Design review of the part built by this model. Coordinates are the model's own, in mm. A direction names the side the tool comes from. Give positions to 0.01 mm unless a question says otherwise; leave off trailing zeros. Loops run counter-clockwise (first coordinate to the right, second up) from the corner with the lowest first, then second, coordinate; pieces in that order, holes last. Notation, with made-up numbers: M 23,36 L 35,36 A22 ccw 35,73 Z; hole C 32.25,-31.75 d7. An arc over 180 degrees is marked long. Answer as CSV lines item,"result".
```python
from build123d import *

# Parameters (mm, degrees)
SKETCH1_R           = 45.25
SKETCH1_R_2         = 38.25
BOSS_EXTRUDE1_DEPTH = 92.5
BOSS_EXTRUDE2_START = -6.35
SKETCH2_R           = 38.25
SKETCH2_R_2         = 36.25
BOSS_EXTRUDE2_DEPTH = 100
CUT_EXTRUDE3_START  = -44
SKETCH6_R           = 39.25
SKETCH6_R_2         = 38.25
CUT_EXTRUDE3_DEPTH  = 44
SKETCH7_R           = 17.5
CUT_EXTRUDE4_DEPTH  = 113.478331247


with BuildPart() as part:
    # Sketch1 → Boss-Extrude1 (new, symmetric)
    with BuildSketch(Plane(origin=(0, 0, 0), x_dir=(1, 0, 0), z_dir=(0, 1, 0))):
        with Locations(Location((0, 0, 0), (0, 0, 270))):
            Circle(SKETCH1_R)
        with Locations(Location((0, 0, 0), (0, 0, 270))):
            Circle(SKETCH1_R_2, mode=Mode.SUBTRACT)
    extrude(amount=BOSS_EXTRUDE1_DEPTH, both=True)

    # Sketch2 → Boss-Extrude2 (add)
    with BuildSketch(Plane.XZ.offset(92.5).offset(BOSS_EXTRUDE2_START)):
        with Locations(Location((0, 0, 0), (0, 0, 270))):
            Circle(SKETCH2_R)
        with Locations(Location((0, 0, 0), (0, 0, 270))):
            Circle(SKETCH2_R_2, mode=Mode.SUBTRACT)
    extrude(amount=-BOSS_EXTRUDE2_DEPTH)

    # Sketch6 → Cut-Extrude3 (cut)
    with BuildSketch(Plane(origin=(0, 92.5, 0), x_dir=(1, 0, 0), z_dir=(0, 1, 0)).offset(CUT_EXTRUDE3_START)):
        with Locations(Location((0, 0, 0), (0, 0, 270))):
            Circle(SKETCH6_R)
        with Locations(Location((0, 0, 0), (0, 0, 90))):
            Circle(SKETCH6_R_2, mode=Mode.SUBTRACT)
    extrude(amount=CUT_EXTRUDE3_DEPTH, mode=Mode.SUBTRACT)

    # Sketch7 → Cut-Extrude4 (cut, through all)
    with BuildSketch(Plane(origin=(0, 0, 0), x_dir=(0, 0, -1), z_dir=(1, 0, 0))):
        with Locations(Location((0, 44.35, 0), (0, 0, 13.717970606))):
            Circle(SKETCH7_R)
    extrude(amount=-CUT_EXTRUDE4_DEPTH, mode=Mode.SUBTRACT)


solid = part.part
```
1. We need section D-D, the plane y = -49. Write out the cut boundary in (x, z).
Answer block:
outline,"C 0,0 d90.5; hole C 0,0 d72.5"
2. We need section A-A, the plane z = 0. Write out the cut boundary in (x, y).
Answer block:
outline,"M -45.25,-92.5 L -38.25,-92.5 L -38.25,-86.15 L -36.25,-86.15 L -36.25,13.85 L -38.25,13.85 L -38.25,26.85 L -45.25,26.85 Z; M -45.25,61.85 L -39.25,61.85 L -39.25,92.5 L -45.25,92.5 Z; M 36.25,-86.15 L 38.25,-86.15 L 38.25,-92.5 L 45.25,-92.5 L 45.25,92.5 L 39.25,92.5 L 39.25,48.5 L 38.25,48.5 L 38.25,13.85 L 36.25,13.85 Z"
3. For P1, Ø2, axis at x = -18.5, y = -19, coming from the +Z side; P2, Ø8, axis at x = 12, y = -70.5, coming from the +Z side; P3, Ø8, axis at y = -26, z = 36, coming from the -X side; P4, Ø23, axis at x = -8, z = -16.5, coming from the -Y side, all flat-tipped, find the tip position at first contact; note any pin that passes through.
Answer block:
P1,"z = 41.73"
P2,"z = 44.54"
P3,"x = -31.99"
P4,"through"
4. For faces 1 (the flat face through (-34, -86.15, -14)), 2 (the cylindrical face through (10.889, -36.85, -34.576)), 3 (the cylindrical face through (-39.538, 26.854, -0.366)), 4 (the flat face through (32.5, 48.5, -20.5)), 5 (the flat face through (37, 92.5, -14)), list the 3-axis set-ups (+Z, -Z, +X, -X, +Y, -Y) from which the entire face can be reached by the end or side of a thin tool; tool diameter is ignored.
Answer block:
face 1,"-Y"
face 2,"+Y, -Y"
face 3,"-X"
face 4,"+Y"
face 5,"+Z, -Z, +X, -X, +Y"
5. The part is to be moulded in two halves that separate along X. For faces 6 (the cylindrical face through (-37.34, -89.37, -8.29)), 7 (the flat face through (37.1, -92.5, -10.3)), 8 (the cylindrical face through (38.155, 1.295, 24.326)), say which applies: pulls with the +X half, pulls with the -X half, needs draft (parallel to the pull), parting line crosses it, or undercut.
Answer block:
face 6,"undercut"
face 7,"needs draft"
face 8,"parting line crosses it"
6. To check wall thickness, follow L1, parallel to X at y = -88, z = 0; L2, parallel to X at y = -13.5, z = 0; L3, parallel to Y at x = 27, z = -26. State the ranges of each line that lie inside material, in increasing order. Write a range as [from, to].
Answer block:
L1,"[-45.25, -38.25], [38.25, 45.25]"
L2,"[-45.25, -36.25], [36.25, 45.25]"
L3,"[-86.15, 13.85]"
7. We need section B-B, the plane x = 0. Write out the cut boundary in (y, z), plus the area to 3 significant figures.
Answer block:
outline,"M -92.5,-45.25 L 92.5,-45.25 L 92.5,-39.25 L 48.5,-39.25 L 48.5,-38.25 L 13.85,-38.25 L 13.85,-36.25 L -86.15,-36.25 L -86.15,-38.25 L -92.5,-38.25 Z; M -92.5,38.25 L -86.15,38.25 L -86.15,36.25 L 13.85,36.25 L 13.85,38.25 L 48.5,38.25 L 48.5,39.25 L 92.5,39.25 L 92.5,45.25 L -92.5,45.25 Z"
area,"2,900 mm²"
8. We need section C-C, the plane z = -30.5. Write out the cut boundary in (x, y).
Answer block:
outline,"M -33.43,-92.5 L -23.08,-92.5 L -23.08,-86.15 L -19.59,-86.15 L -19.59,13.85 L -23.08,13.85 L -23.08,48.5 L -24.7,48.5 L -24.7,92.5 L -33.43,92.5 Z; M 19.59,-86.15 L 23.08,-86.15 L 23.08,-92.5 L 33.43,-92.5 L 33.43,92.5 L 24.7,92.5 L 24.7,48.5 L 23.08,48.5 L 23.08,13.85 L 19.59,13.85 Z"
